For this review, take the finished solid that the model builds, in its own axes (mm). A direction names the side the tool comes from. Coordinates: 2 decimals unless noted, no trailing zeros. Loops run counter-clockwise (first coordinate to the right, second up) from the corner with the lowest first, then second, coordinate; pieces in that order, holes last. Notation, with made-up numbers: (81, 76.25) -> (104, 76.25) arc R22 cw to (104, 109.25) -> close; hole circle Ø7 at (85.25, -1.5). An arc over 180 degrees is marked (long way). Answer in a Markdown table with one row per item.
from build123d import *

# Parameters (mm, degrees)
SKETCH1_R                                      = 1.35
SKETCH1_R_2                                    = 6
SKETCH1_R_3                                    = 3.1
BOSS_EXTRUDE1_DEPTH                            = 4
CSK_FOR_M2_5_FLAT_HEAD_MACHINE_SCREW1_AT_COUNT = 2
CSK_FOR_M2_5_FLAT_HEAD_MACHINE_SCREW1_AT_PITCH = 43
CSK_FOR_M2_5_FLAT_HEAD_MACHINE_SCREW_2_COUNT   = 2
CSK_FOR_M2_5_FLAT_HEAD_MACHINE_SCREW_2_PITCH   = 60.811183182
CSK_FOR_M2_5_FLAT_HEAD_MACHINE_SCREW_3_COUNT   = 2
CSK_FOR_M2_5_FLAT_HEAD_MACHINE_SCREW_3_PITCH   = 43


with BuildPart() as part:
    # Sketch1 → Boss-Extrude1 (new body)
    with BuildSketch(Plane.XY):
        with BuildLine():
            Line((-27.744938631, 6), (27.744938631, 6))
            Line((27.744938631, 6), (27.744938631, 16.75))
            ThreePointArc((27.744938631, 16.75), (24.524595568, 24.52459576), (16.749999729, 27.744938631))
            Line((16.749999729, 27.744938631), (-16.75, 27.744938631))
            ThreePointArc((-16.75, 27.744938631), (-24.524595664, 24.524595664), (-27.744938631, 16.75))
            Line((-27.744938631, 16.75), (-27.744938631, 6))
        make_face()
        with Locations((-21.5, 21.5)):
            Circle(SKETCH1_R, mode=Mode.SUBTRACT)
        with Locations((21.5, 21.5)):
            Circle(SKETCH1_R, mode=Mode.SUBTRACT)
        Polygon((-27.744938631, -6), (27.744938631, -6), (27.744938631, 0), (27.744938631, 6), (-27.744938631, 6), (-27.744938631, 0), align=None)
        with BuildLine():
            Line((-16.749999529, -27.744938631), (16.75, -27.744938631))
            ThreePointArc((16.75, -27.744938631), (24.524595836, -24.524595492), (27.744938631, -16.749999513))
            Line((27.744938631, -16.749999513), (27.744938631, -6))
            Line((27.744938631, -6), (-27.744938631, -6))
            Line((-27.744938631, -6), (-27.744938631, -16.75))
            ThreePointArc((-27.744938631, -16.75), (-24.524595498, -24.524595831), (-16.749999529, -27.744938631))
        make_face()
        with Locations((-21.5, -21.5)):
            Circle(SKETCH1_R, mode=Mode.SUBTRACT)
        with Locations((21.5, -21.5)):
            Circle(SKETCH1_R, mode=Mode.SUBTRACT)
        with BuildLine():
            Line((-33.744938608, -6), (-27.744938631, -6))
            Line((-27.744938631, -6), (-27.744938631, 0))
            ThreePointArc((-27.744938631, 0), (-29.502297935, -4.242640679), (-33.744938608, -6))
        make_face()
        with BuildLine():
            ThreePointArc((-33.744938605, 6), (-29.502297934, 4.242640678), (-27.744938631, 0))
            Line((-27.744938631, 0), (-27.744938631, 6))
            Line((-27.744938631, 6), (-33.744938605, 6))
        make_face()
        with Locations((-33.744938631, 0)):
            Circle(SKETCH1_R_2)
        with Locations((-33.744938631, 0)):
            Circle(SKETCH1_R_3, mode=Mode.SUBTRACT)
        with BuildLine():
            Line((27.744938631, 6), (27.744938631, 0))
            ThreePointArc((27.744938631, 0), (29.502297943, 4.242640687), (33.744938631, 6))
            Line((33.744938631, 6), (27.744938631, 6))
        make_face()
        with BuildLine():
            Line((27.744938631, 0), (27.744938631, -6))
            Line((27.744938631, -6), (33.744938631, -6))
            ThreePointArc((33.744938631, -6), (29.502297943, -4.242640687), (27.744938631, 0))
        make_face()
        with Locations((33.744938631, 0)):
            Circle(SKETCH1_R_2)
        with Locations((33.744938631, 0)):
            Circle(SKETCH1_R_3, mode=Mode.SUBTRACT)
    extrude(amount=-BOSS_EXTRUDE1_DEPTH)

    # Sketch3 → CSK for M2.5 Flat Head Machine Screw1 (revolve, cut)
    with BuildSketch(Plane(origin=(21.5, 21.5, -4), x_dir=(0, 1, 0), z_dir=(1, 0, 0))):
        Polygon((0, 0), (0, 4), (1.25, 4), (1.25, 1.55), (2.5, 0.3), (2.5, 0), align=None)
    csk_for_m2_5_flat_head_machine_screw1 = revolve(axis=Axis((21.5, 21.5, -10.35), (0, 0, 1)), mode=Mode.SUBTRACT)

    # CSK for M2.5 Flat Head Machine Screw1 at: CSK for M2.5 Flat Head Machine Screw1 ×2
    with Locations(*[(-i * CSK_FOR_M2_5_FLAT_HEAD_MACHINE_SCREW1_AT_PITCH, 0, 0) for i in range(1, CSK_FOR_M2_5_FLAT_HEAD_MACHINE_SCREW1_AT_COUNT)]):
        add(csk_for_m2_5_flat_head_machine_screw1, mode=Mode.SUBTRACT)

    # CSK for M2.5 Flat Head Machine Screw 2: CSK for M2.5 Flat Head Machine Screw1 ×2
    with Locations(*[Vector(-0.707106781, -0.707106781, 0) * (i * CSK_FOR_M2_5_FLAT_HEAD_MACHINE_SCREW_2_PITCH) for i in range(1, CSK_FOR_M2_5_FLAT_HEAD_MACHINE_SCREW_2_COUNT)]):
        add(csk_for_m2_5_flat_head_machine_screw1, mode=Mode.SUBTRACT)

    # CSK for M2.5 Flat Head Machine Screw 3: CSK for M2.5 Flat Head Machine Screw1 ×2
    with Locations(*[(0, -i * CSK_FOR_M2_5_FLAT_HEAD_MACHINE_SCREW_3_PITCH, 0) for i in range(1, CSK_FOR_M2_5_FLAT_HEAD_MACHINE_SCREW_3_COUNT)]):
        add(csk_for_m2_5_flat_head_machine_screw1, mode=Mode.SUBTRACT)


solid = part.part
Item 1: Take a section at B-B, the plane y = 0. State the section outline as (x, z) points.
Worked answers:
| item | result |
|---|---|
| outline | (-39.74, -4) -> (-36.84, -4) -> (-36.84, 0) -> (-39.74, 0) -> close; (-30.64, -4) -> (30.64, -4) -> (30.64, 0) -> (-30.64, 0) -> close; (36.84, -4) -> (39.74, -4) -> (39.74, 0) -> (36.84, 0) -> close |
Item 2: Insertion check: pin 1 (1.2 mm diameter, centred on y = 9.5, z = -2, fed in from +X); pin 2 (3 mm diameter, centred on x = 21.5, y = 21.5, fed in from -Z); pin 3 (1.5 mm diameter, centred on y = -22, z = -2.5, fed in from -X). Each pin has a flat end and moves straight along its axis. Give the tip position at first contact, or say it passes through.
Worked answers:
| item | result |
|---|---|
| pin 1 | x = 27.74 |
| pin 2 | z = -2.7 |
| pin 3 | x = -26.78 |
Item 3: Take a section at C-C, the plane x = -21.5. State the section outline as (y, z) points, and give its area (3 significant figures).
Worked answers:
| item | result |
|---|---|
| outline | (-26.67, -4) -> (-24, -4) -> (-24, -3.7) -> (-22.85, -2.55) -> (-22.85, 0) -> (-26.67, 0) -> close; (-20.15, -2.55) -> (-19, -3.7) -> (-19, -4) -> (19, -4) -> (19, -3.7) -> (20.15, -2.55) -> (20.15, 0) -> (-20.15, 0) -> close; (22.85, -2.55) -> (24, -3.7) -> (24, -4) -> (26.67, -4) -> (26.67, 0) -> (22.85, 0) -> close |
| area | 188 mm² |
Item 4: For faces 4 (the flat face through (-1, 0, -4)), 5 (the flat face through (27.745, 11, -2)), 6 (the cylindrical face through (-23.19, 19.66, -3.85)), 7 (the flat face through (31, -6, -2)), 8 (the flat face through (-31, -6, -2)), list the 3-axis set-ups (+Z, -Z, +X, -X, +Y, -Y) from which the entire face can be reached by the end or side of a thin tool; tool diameter is ignored.
Worked answers:
| item | result |
|---|---|
| face 4 | -Z, +X, -X, +Y, -Y |
| face 5 | +Z, -Z, +X, +Y |
| face 6 | -Z |
| face 7 | +Z, -Z, +X, -Y |
| face 8 | +Z, -Z, -X, -Y |
Item 5: For L1, parallel to Y at x = 21.5, z = -0.75; L2, parallel to X at y = -1.5, z = -3.75; L3, parallel to X at y = -2.5, z = -2.95, list the stretches that pass through material, from the lowest coordinate up.
Worked answers:
| item | result |
|---|---|
| L1 | -26.67 to -22.85, -20.15 to 20.15, 22.85 to 26.67 |
| L2 | -39.55 to -36.46, -31.03 to 31.03, 36.46 to 39.55 |
| L3 | -39.2 to -35.58, -31.91 to 31.91, 35.58 to 39.2 |
Item 6: Take a section at A-A, the plane z = -1.85. State the section outline as (x, y) points.
Worked answers:
| item | result |
|---|---|
| outline | (-33.74, -6) -> (-27.74, -6) -> (-27.74, -16.75) arc R10.99 ccw to (-16.75, -27.74) -> (16.75, -27.74) arc R10.99 ccw to (27.74, -16.75) -> (27.74, -6) -> (33.74, -6) arc R6 ccw to (33.74, 6) -> (27.74, 6) -> (27.74, 16.75) arc R10.99 ccw to (16.75, 27.74) -> (-16.75, 27.74) arc R10.99 ccw to (-27.74, 16.75) -> (-27.74, 6) -> (-33.74, 6) arc R6 ccw to start; hole circle Ø6.2 at (-33.74, 0); hole circle Ø2.7 at (-21.5, -21.5); hole circle Ø2.7 at (-21.5, 21.5); hole circle Ø2.7 at (21.5, -21.5); hole circle Ø2.7 at (21.5, 21.5); hole circle Ø6.2 at (33.74, 0) |
Item 7: The part is to be moulded in two halves that separate along X. For faces 1 (the flat face through (-27.745, 11, -2)), 2 (the cylindrical face through (-19.06, -22.04, -3.85)), 3 (the flat face through (31, 6, -2)), say which applies: +X half, -X half, draft (parallel to the pull), parting line (faces both ways), or undercut.
Worked answers:
| item | result |
|---|---|
| face 1 | -X half |
| face 2 | undercut |
| face 3 | draft |
